Part model, mm, in its own coordinate system. A direction names the side the tool comes from. Round coordinates to 2 decimals unless told otherwise and drop trailing zeros. Loops run counter-clockwise (first coordinate to the right, second up) from the corner with the lowest first, then second, coordinate; pieces in that order, holes last. Notation, with made-up numbers: (85.25, -21.5) -> (142.25, -21.5) arc R33 ccw to (142.25, 7.5) -> close; hole circle Ø5 at (51, 12.5). An arc over 180 degrees is marked (long way). Use a Markdown table: item, result. Add a question column.
Item 1: Cut at C-C, the plane x = -81.5. List the corners of the cut face in (y, z), plus the area to 3 significant figures.
Item 2: Cut at B-B, the plane y = 71. List the corners of the cut face in (x, z), plus the area to 3 significant figures.
Item 3: Probe line 1 (Y direction, x = 10.5, z = 43); line 2 (Y direction, x = 61, z = 15.5); line 3 (Z direction, x = -65.5, y = 44). List the from-to ranges inside material, lowest first. Write a range as [from, to].
Item 4: Which spindle directions (+Z, -Z, +X, -X, +Y, -Y) get a long thin tool onto all of the face, cutting with end or side? Do faces 1 (the face through (38.66, 56.57, -18.27)), 2 (the face through (-95, 32, 1)), 3 (the face through (-53, 62, -75)). Say none if no direction does.
Item 5: Flat gauge pins, fed straight in: pin 1 (5 mm diameter, centred on x = -6.5, z = 27, fed in from -Y); pin 2 (6 mm diameter, centred on x = 48, y = 32.5, fed in from +Z); pin 3 (13.5 mm diameter, centred on y = 67, z = -2.5, fed in from +X); pin 4 (3.5 mm diameter, centred on x = -66.5, z = -73.5, fed in from +Y). Where does each tip first touch, or does it go through?
Item 6: Cut at A-A, the plane x = 2. List the corners of the cut face in (y, z), plus the area to 3 significant figures.
```python
from build123d import *

# Parameters (mm, degrees)
SKETCH1_W           = 190
SKETCH1_H           = 156
BOSS_EXTRUDE1_DEPTH = 84
CUT_EXTRUDE1_DEPTH  = 222.900878772
CUT_EXTRUDE2_DEPTH  = 104
FILLET1_R           = 50
FILLET2_R           = 10
FILLET3_R           = 10


with BuildPart() as part:
    # Sketch1 → Boss-Extrude1 (new body)
    with BuildSketch(Plane(origin=(0, 0, 0), x_dir=(1, 0, 0), z_dir=(0, 1, 0))):
        Rectangle(SKETCH1_W, SKETCH1_H)
    extrude(amount=BOSS_EXTRUDE1_DEPTH)

    # Sketch2 → Cut-Extrude1 (cut, through all)
    with BuildSketch(Plane.ZY.offset(95)):
        Polygon((-78, 84), (-78, 62), (-71, 62), (-59.118583078, 84), align=None)
        Polygon((78, 84), (-59.118583078, 84), (45.881416922, 60), (75, 38), (78, 10), align=None)
    extrude(amount=-CUT_EXTRUDE1_DEPTH, mode=Mode.SUBTRACT)

    # Sketch3 → Cut-Extrude2 (cut)
    with BuildSketch(Plane(origin=(95, 0, 0), x_dir=(0, 0, -1), z_dir=(1, 0, 0))):
        Polygon((-54, 50), (-75, 38), (-45.881416922, 60), (59.118583078, 84), (71, 62), (78, 62), align=None)
    extrude(amount=-CUT_EXTRUDE2_DEPTH, mode=Mode.SUBTRACT)

    # Fillet1
    fillet1_edges = [part.edges().sort_by_distance(p)[0] for p in [
        (43, 50, 54),
    ]]
    fillet(fillet1_edges, radius=FILLET1_R)

    # Fillet2
    fillet2_edges = [part.edges().sort_by_distance(p)[0] for p in [
        (-52, 84, -59.118583078),
    ]]
    fillet(fillet2_edges, radius=FILLET2_R)

    # Fillet3
    fillet3_edges = [part.edges().sort_by_distance(p)[0] for p in [
        (-52, 60, 45.881416922),
        (95, 56.49247454, -17.417219937),
        (95, 41.301222931, 69.22285987),
        (95, 48.884092571, 53.64880539),
    ]]
    fillet(fillet3_edges, radius=FILLET3_R)


solid = part.part
```
A:
| question | item | result |
|---|---|---|
| 1 | outline | (0, -78) -> (62, -78) -> (62, -71) -> (77.31, -62.73) arc R10 ccw to (82.31, -51.71) -> (60.48, 43.79) arc R10 ccw to (58.71, 47.59) -> (38, 75) -> (10, 78) -> (0, 78) -> close |
| 1 | area | 10,300 mm^2 |
| 2 | outline | (-95, -66.14) -> (-9, -66.14) -> (-9, -2.24) -> (-95, -2.24) -> close |
| 2 | area | 5,500 mm^2 |
| 3 | line 1 | y = [0, 51] |
| 3 | line 2 | y = [0, 53.5] |
| 3 | line 3 | z = [-78, 67.06] |
| 4 | face 1 | +Z, +X, +Y |
| 4 | face 2 | +Z, -Z, -X, +Y, -Y |
| 4 | face 3 | -Z, +X, -X, +Y |
| 5 | pin 1 | stops at y = 0 |
| 5 | pin 2 | stops at z = 75.91 |
| 5 | pin 3 | stops at x = -9 |
| 5 | pin 4 | stops at y = 62 |
| 6 | outline | (0, -78) -> (62, -78) -> (50.98, 43.17) arc R50 ccw to (44.6, 63.45) -> (38, 75) -> (10, 78) -> (0, 78) -> close |
| 6 | area | 8,380 mm^2 |
